Part model, mm, in its own coordinate system. Face numbers are marked on the shaded views. A direction names the side the tool comes from. Give positions to 0.01 mm unless a question says otherwise; leave off trailing zeros. Write each loop counter-clockwise with the first axis right and the second up, starting at its lowest first coordinate (ties: lowest second). Pieces come first, ordered by that corner, then holes.
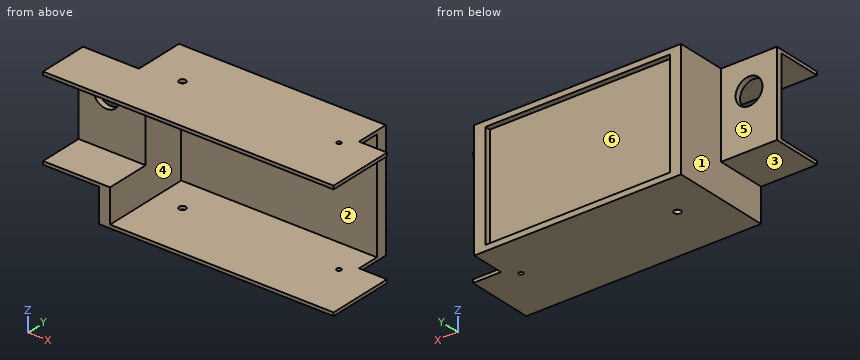
from build123d import *

# Parameters (mm, degrees)
SKETCH_2_W          = 210
SKETCH_2_H          = 105
EXTRUDE_1_DEPTH     = 90
SKETCH_4_W          = 165
SKETCH_4_H          = 95
CUT_EXTRUDE_1_DEPTH = 5
SKETCH_5_W          = 99
SKETCH_5_H          = 80
CUT_EXTRUDE_2_DEPTH = 200
SKETCH_6_W          = 75
SKETCH_6_H          = 45
EXTRUDE_2_DEPTH     = 50
SKETCH_7_W          = 69
SKETCH_7_H          = 40
CUT_EXTRUDE_3_DEPTH = 281.100428418
SKETCH_8_R          = 12
CUT_EXTRUDE_4_DEPTH = 170.724040725
SKETCH_9_R          = 3
SKETCH_9_R_2        = 2
CUT_EXTRUDE_5_DEPTH = 208.725780778
SKETCH_11_W         = 25
SKETCH_11_H         = 105
CUT_EXTRUDE_6_DEPTH = 30


with BuildPart() as part:
    # 草图2 → 凸台-拉伸1 (new body)
    with BuildSketch(Plane(origin=(0, 0, 0), x_dir=(1, 0, 0), z_dir=(0, 1, 0))):
        Rectangle(SKETCH_2_W, SKETCH_2_H)
    extrude(amount=EXTRUDE_1_DEPTH)

    # 草图4 → 切除-拉伸1 (cut)
    with BuildSketch(Plane(origin=(0, 90, 0), x_dir=(1, 0, 0), z_dir=(0, 1, 0))):
        with Locations((-12.5, 0)):
            Rectangle(SKETCH_4_W, SKETCH_4_H)
    extrude(amount=-CUT_EXTRUDE_1_DEPTH, mode=Mode.SUBTRACT)

    # 草图5 → 切除-拉伸2 (cut)
    with BuildSketch(Plane(origin=(105, 0, 0), x_dir=(0, 0, -1), z_dir=(1, 0, 0))):
        with Locations((0, 40)):
            Rectangle(SKETCH_5_W, SKETCH_5_H)
    extrude(amount=-CUT_EXTRUDE_2_DEPTH, mode=Mode.SUBTRACT)

    # 草图6 → 凸台-拉伸2 (add)
    with BuildSketch(Plane.ZY.offset(105)):
        with Locations((15, 22.5)):
            Rectangle(SKETCH_6_W, SKETCH_6_H)
    extrude(amount=EXTRUDE_2_DEPTH)

    # 草图7 → 切除-拉伸3 (cut, through all)
    with BuildSketch(Plane.ZY.offset(155)):
        with Locations((15, 20)):
            Rectangle(SKETCH_7_W, SKETCH_7_H)
    extrude(amount=-CUT_EXTRUDE_3_DEPTH, mode=Mode.SUBTRACT)

    # 草图8 → 切除-拉伸4 (cut, through all)
    with BuildSketch(Plane(origin=(0, 45, 0), x_dir=(1, 0, 0), z_dir=(0, 1, 0))):
        with Locations(Location((-130, -25.5, 0), (0, 0, 270))):
            Circle(SKETCH_8_R)
    extrude(amount=-CUT_EXTRUDE_4_DEPTH, mode=Mode.SUBTRACT)

    # 草图9 → 切除-拉伸5 (cut, through all)
    with BuildSketch(Plane.XY.offset(52.5)):
        with Locations((-70, 50)):
            Circle(SKETCH_9_R)
        with Locations((70, 50)):
            Circle(SKETCH_9_R_2)
    extrude(amount=-CUT_EXTRUDE_5_DEPTH, mode=Mode.SUBTRACT)

    # 草图11 → 切除-拉伸6 (cut)
    with BuildSketch(Plane(origin=(0, 90, 0), x_dir=(1, 0, 0), z_dir=(0, 1, 0))):
        with Locations((92.5, 0)):
            Rectangle(SKETCH_11_W, SKETCH_11_H)
    extrude(amount=-CUT_EXTRUDE_6_DEPTH, mode=Mode.SUBTRACT)


solid = part.part
1) Drill centre lines: L1, parallel to Z at x = -32, y = 75.5; L2, parallel to Y at x = -70, z = 51.7; L3, parallel to Y at x = 70, z = -51.55. Where is each one in solid material? Low to high.
Check result:
L1: z = -52.5 to -49.5, 49.5 to 52.5
L2: y = 0 to 47, 53 to 90
L3: y = 0 to 48, 52 to 90
2) Saw through at D-D (y = 66.5). Write the cut outline in (x, z).
Check result:
outline: (-105, -52.5) - (80, -52.5) - (80, -49.5) - (-95, -49.5) - (-95, 49.5) - (80, 49.5) - (80, 52.5) - (-105, 52.5) - close
3) Saw through at B-B (z = 25.5). Write the cut outline in (x, y).
Check result:
outline: (-155, 40) - (-142, 40) - (-142, 45) - (-155, 45) - close; (-118, 40) - (-95, 40) - (-95, 80) - (80, 80) - (80, 90) - (70, 90) - (70, 85) - (-95, 85) - (-95, 90) - (-105, 90) - (-105, 45) - (-118, 45) - close
4) Flat gauge pins, fed straight in: P1, Ø13.5, axis at x = -138.5, y = 19, coming from the -Z side; P2, Ø4, axis at y = 70, z = 18, coming from the -X side; P3, Ø1.5, axis at x = 62.5, z = -4, coming from the +Y side. Where does each tip first touch, or does it go through?
Check result:
P1: stops at z = -22.5
P2: stops at x = -105
P3: stops at y = 85
5) 3-axis set-ups, long thin cutter, end or side, ignore diameter. For the marked faces 4, 5 and 6: which of +Z, -Z, +X, -X, +Y, -Y reach the whole face in a straight line?
Check result:
face 4: +X, -Y
face 5: +Z, -Z, -X, +Y
face 6: +Y
6) Mould opens along Z. For the marked faces 1, 2 and 3 say: +Z half, -Z half, draft (parallel to the pull), parting line (faces both ways), or undercut.
Check result:
face 1: draft
face 2: undercut
face 3: -Z half
7) Saw through at A-A (x = -130). Write the cut outline in (y, z), and give its area (3 significant figures).
Check result:
outline: (0, -22.5) - (45, -22.5) - (45, 13.5) - (40, 13.5) - (40, -19.5) - (0, -19.5) - close; (0, 49.5) - (40, 49.5) - (40, 37.5) - (45, 37.5) - (45, 52.5) - (0, 52.5) - close
area: 495 mm2
8) Saw through at C-C (x = -70). Write the cut outline in (y, z), and give its area (3 significant figures).
Check result:
outline: (0, -52.5) - (47, -52.5) - (47, -49.5) - (0, -49.5) - close; (0, 49.5) - (47, 49.5) - (47, 52.5) - (0, 52.5) - close; (53, -52.5) - (90, -52.5) - (90, -47.5) - (85, -47.5) - (85, 47.5) - (90, 47.5) - (90, 52.5) - (53, 52.5) - (53, 49.5) - (80, 49.5) - (80, -49.5) - (53, -49.5) - close
area: 1,020 mm2
